Answer from the drawing. Dimensions are ordinates in mm from the lowest x, y and z of the part. A direction names the side the tool comes from. Give positions to 0.01 mm unless a question says otherwise; leave off trailing zeros. Loops run counter-clockwise (first coordinate to the right, second up) from the corner with the lowest first, then second, coordinate; pieces in that order, holes last.
(1) Straight lines are drawn through the part: probe 1 along Y at (x, z) = (66, 13.55); probe 2 along Y at (x, z) = (41.5, 14.25); probe 3 along X at (y, z) = (39.5, 6.5). For each, find the intervals that lie inside material, in ascending order.
(2) Determine the mould class of the marked faces 3, 4, 5 and 6 for opening direction X: pulls with the +X half, pulls with the -X half, needs draft (parallel to the pull), parting line crosses it, or undercut.
(3) Find section A-A, the plane z = 13. State how many separate pieces and enclosed holes the cut face has, then the cut area to 3 significant figures.
(4) Find section C-C, the plane z = 2.25. Write down the section's boundary in (x, y).
(5) Which of the six approach directions +Z, -Z, +X, -X, +Y, -Y give full straight-line access (tool end or side, diameter ignored) to the marked faces 1 and 2?
(6) Find section D-D, the plane y = 6.5. Write down the section's boundary in (x, z).
(7) Find section B-B, the plane x = 23. Write down the section's boundary in (y, z), then the cut area to 3 significant figures.
(8) Each of these flat-tipped pins is pushed along its axis until it touches: P1, Ø2, axis at x = 8, y = 6, coming from the -Z side; P2, Ø12, axis at x = 19.5, y = 24.5, coming from the -Z side. Where does it stop, or does it pass through?
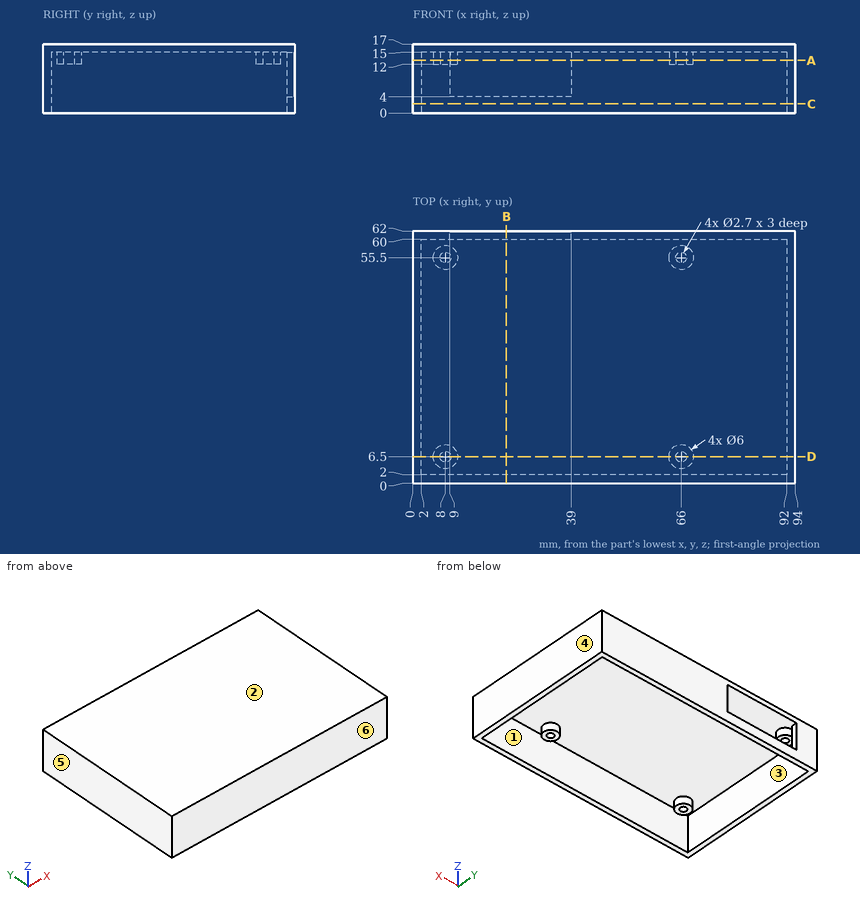
Entries:
1. probe 1: y = 0 to 2, 3.5 to 5.15, 7.85 to 9.5, 52.5 to 54.15, 56.85 to 58.5, 60 to 62
1. probe 2: y = 0 to 2, 60 to 62
1. probe 3: x = 0 to 2, 92 to 94
2. face 3: undercut
2. face 4: pulls with the +X half
2. face 5: pulls with the -X half
2. face 6: needs draft
3. separate pieces: 5
3. enclosed holes: 4
3. area: 638 mm2
4. outline: (0, 0) - (94, 0) - (94, 62) - (0, 62) - close; hole (2, 2) - (92, 2) - (92, 60) - (2, 60) - close
5. face 1: -Z
5. face 2: +Z, +X, -X, +Y, -Y
6. outline: (0, 0) - (2, 0) - (2, 15) - (5, 15) - (5, 12) - (6.65, 12) - (6.65, 15) - (9.35, 15) - (9.35, 12) - (11, 12) - (11, 15) - (63, 15) - (63, 12) - (64.65, 12) - (64.65, 15) - (67.35, 15) - (67.35, 12) - (69, 12) - (69, 15) - (92, 15) - (92, 0) - (94, 0) - (94, 17) - (0, 17) - close
7. outline: (0, 0) - (2, 0) - (2, 15) - (62, 15) - (62, 17) - (0, 17) - close; (60, 0) - (62, 0) - (62, 4) - (60, 4) - close
7. area: 162 mm2
8. P1: stops at z = 12
8. P2: stops at z = 15
